Model file for the job. Use its own axes, mm. Give positions to 0.01 mm unless a question says otherwise; leave off trailing zeros. Loops run counter-clockwise (first coordinate to the right, second up) from the corner with the lowest first, then second, coordinate; pieces in that order, holes last. Notation, with made-up numbers: (-4, 24) - (50, 24) arc R19 cw to (50, 55) - close; hole circle Ø9 at (66, -18). An arc over 180 degrees is marked (long way). Use a Markdown table: item, result.
from build123d import *

# Parameters (mm, degrees)
SKETCH1_R           = 4
SKETCH1_R_2         = 1
BOSS_EXTRUDE1_DEPTH = 3


with BuildPart() as part:
    # Sketch1 → Boss-Extrude1 (new body)
    with BuildSketch(Plane(origin=(0, 0, 0), x_dir=(1, 0, 0), z_dir=(0, 1, 0))):
        with BuildLine():
            ThreePointArc((-35.678871137, -35.738888545), (50.325579201, 4.193575813), (-41.101893418, 29.340830893))
            ThreePointArc((-41.101893418, 29.340830893), (-13.951645719, -1.162575473), (-35.678871137, -35.738888545))
        make_face()
        with Locations(Location((0, 0, 0), (0, 0, 270))):
            Circle(SKETCH1_R, mode=Mode.SUBTRACT)
        with Locations(Location((-6.318484242, 0, 0), (0, 0, 270))):
            Circle(SKETCH1_R_2, mode=Mode.SUBTRACT)
        with Locations(Location((0, 6.8, 0), (0, 0, 270))):
            Circle(SKETCH1_R_2, mode=Mode.SUBTRACT)
        with Locations(Location((6.8, 0, 0), (0, 0, 270))):
            Circle(SKETCH1_R_2, mode=Mode.SUBTRACT)
        with Locations(Location((0, -6.8, 0), (0, 0, 270))):
            Circle(SKETCH1_R_2, mode=Mode.SUBTRACT)
    extrude(amount=BOSS_EXTRUDE1_DEPTH)


solid = part.part
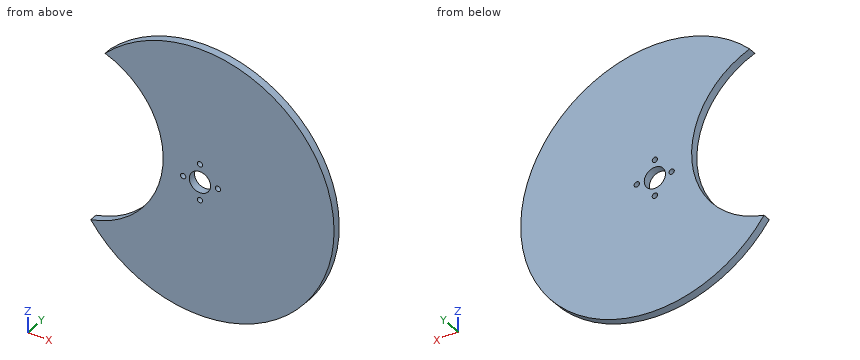
(1) Slice it at C-C, the plane z = -42. Write the cut outline in (x, y), plus the area to 3 significant figures.
Computed:
| item | result |
|---|---|
| outline | (-28.04, 0) - (28.04, 0) - (28.04, 3) - (-28.04, 3) - close |
| area | 168 mm² |
(2) Slice it at A-A, the plane x = -25. Write the cut outline in (y, z), plus the area to 3 significant figures.
Computed:
| item | result |
|---|---|
| outline | (0, -43.88) - (3, -43.88) - (3, -21.21) - (0, -21.21) - close; (0, 29.18) - (3, 29.18) - (3, 43.88) - (0, 43.88) - close |
| area | 112 mm² |
(3) Slice it at B-B, the plane y = 2.1. Write the cut outline in (x, z), plus the area to 3 significant figures.
Computed:
| item | result |
|---|---|
| outline | (-41.1, -29.34) arc R50.5 ccw (long way) to (-35.68, 35.74) arc R34 cw to start; hole circle Ø2 at (-6.32, 0); hole circle Ø8 at (0, 0); hole circle Ø2 at (0, -6.8); hole circle Ø2 at (0, 6.8); hole circle Ø2 at (6.8, 0) |
| area | 6,230 mm² |
(4) Pin check, flat tips, straight feed: P1, Ø1.8, axis at x = 0, z = 6.8, coming from the +Y side; P2, Ø3, axis at x = 0, z = -6.8, coming from the -Y side; P3, Ø1.5, axis at y = 1.5, z = 15.5, coming from the +X side. Stop position of each tip, or through.
Computed:
| item | result |
|---|---|
| P1 | through |
| P2 | y = 0 |
| P3 | x = 48.3 |
(5) Slice it at D-D, the plane x = 30.5. Write the cut outline in (y, z).
Computed:
| item | result |
|---|---|
| outline | (0, -40.25) - (3, -40.25) - (3, 40.25) - (0, 40.25) - close |
(6) Drill centre lines: probe 1 along X at (y, z) = (1.55, 0); probe 2 along Z at (x, y) = (-31, 0.6); probe 3 along Z at (x, y) = (-22.5, 1.75). Where is each one in solid material? Low to high. Write a range as [from, to].
Computed:
| item | result |
|---|---|
| probe 1 | [-14.07, -7.32], [-5.32, -4], [4, 5.8], [7.8, 50.5] |
| probe 2 | [-39.87, -25.55], [33.53, 39.87] |
| probe 3 | [-45.21, -18.69], [26.66, 45.21] |
